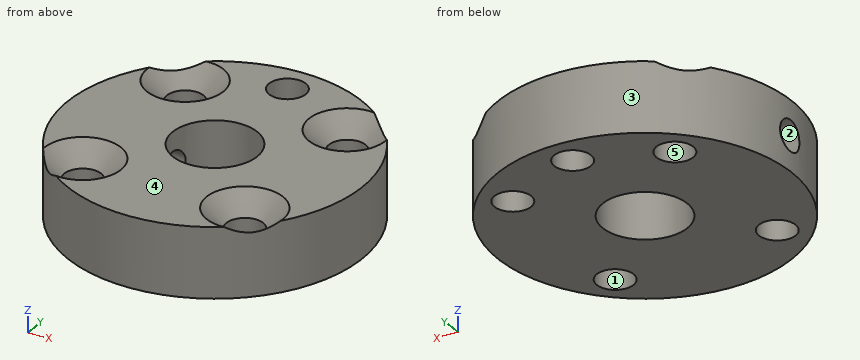
```python
from build123d import *

# Parameters (mm, degrees)
SKETCH2_R                                       = 20
BOSS_EXTRUDE1_DEPTH                             = 9.5
CSK_FOR_M5_FLAT_HEAD_MACHINE_SCREW1_D           = 5
CSK_FOR_M5_FLAT_HEAD_MACHINE_SCREW1_CSINK_D     = 10.4
CSK_FOR_M5_FLAT_HEAD_MACHINE_SCREW1_CSINK_ANGLE = 90
SKETCH5_R                                       = 2.5
CUT_EXTRUDE1_DEPTH                              = 30.837057662
SKETCH6_R                                       = 5.75
CUT_EXTRUDE2_DEPTH                              = 30.837057662
SKETCH8_R                                       = 2.1
CUT_EXTRUDE3_DEPTH                              = 30.837057662


with BuildPart() as part:
    # Sketch2 → Boss-Extrude1 (new body)
    with BuildSketch(Plane.XY):
        Circle(SKETCH2_R)
    extrude(amount=BOSS_EXTRUDE1_DEPTH)

    # CSK for M5 Flat Head Machine Screw1 (through all)
    with Locations(Plane.XY.offset(9.5)):
        with Locations((-11.136931804, 11.136931804), (11.136931804, 11.136931804), (11.136931804, -11.136931804), (-11.136931804, -11.136931804)):
            CounterSinkHole(CSK_FOR_M5_FLAT_HEAD_MACHINE_SCREW1_D / 2, CSK_FOR_M5_FLAT_HEAD_MACHINE_SCREW1_CSINK_D / 2, counter_sink_angle=CSK_FOR_M5_FLAT_HEAD_MACHINE_SCREW1_CSINK_ANGLE)

    # Sketch5 → Cut-Extrude1 (cut, through all)
    with BuildSketch(Plane.XY.offset(9.5)):
        with Locations((0, 15.75)):
            Circle(SKETCH5_R)
    extrude(amount=-CUT_EXTRUDE1_DEPTH, mode=Mode.SUBTRACT)

    # Sketch6 → Cut-Extrude2 (cut, through all)
    with BuildSketch(Plane.XY.offset(9.5)):
        Circle(SKETCH6_R)
    extrude(amount=-CUT_EXTRUDE2_DEPTH, mode=Mode.SUBTRACT)

    # Sketch8 → Cut-Extrude3 (cut, through all)
    with BuildSketch(Plane(origin=(0, 0, 0), x_dir=(0, 0, -1), z_dir=(1, 0, 0))):
        with Locations((-4.75, 0)):
            Circle(SKETCH8_R)
    extrude(amount=-CUT_EXTRUDE3_DEPTH, mode=Mode.SUBTRACT)


solid = part.part
```
Design review of the part built by this model. Coordinates are the model's own, in mm. Face numbers are marked on the shaded views. A direction names the side the tool comes from. Coordinates: 2 decimals unless noted, no trailing zeros. Loops run counter-clockwise (first coordinate to the right, second up) from the corner with the lowest first, then second, coordinate; pieces in that order, holes last.
Q1. We need section D-D on x = 4.5. State the section outline as (y, z) points, and give its area (3 significant figures).
Reported:
outline: (-19.49, 0) - (-3.58, 0) - (-3.58, 9.5) - (-19.49, 9.5) - close; (3.58, 0) - (19.49, 0) - (19.49, 9.5) - (3.58, 9.5) - close
area: 302 mm2
Q2. To check wall thickness, follow line 1 (Y direction, x = 0, z = 3); line 2 (X direction, y = -11, z = 6); line 3 (X direction, y = -13, z = 1.5). State the ranges of each line that lie inside material, in increasing order.
Reported:
line 1: y = -20 to -5.75, 5.75 to 13.25, 18.25 to 20
line 2: x = -16.7 to -13.63, -8.64 to 8.64, 13.63 to 16.7
line 3: x = -15.2 to -12.8, -9.47 to 9.47, 12.8 to 15.2
Q3. Tool access review of the marked faces 1 and 2: name each direction out of +Z, -Z, +X, -X, +Y, -Y from which nothing blocks a thin tool from reaching the whole face with its end or side.
Reported:
face 1: +Z, -Z
face 2: -X
Q4. We need section B-B on x = 0. State the section outline as (y, z) points.
Reported:
outline: (-20, 0) - (-5.75, 0) - (-5.75, 9.5) - (-20, 9.5) - close; (5.75, 0) - (13.25, 0) - (13.25, 9.5) - (5.75, 9.5) - close; (18.25, 0) - (20, 0) - (20, 9.5) - (18.25, 9.5) - close
Q5. We need section C-C on z = 4.75. State the section outline as (x, y) points.
Reported:
outline: (-19.89, -2.1) arc R20 ccw (long way) to (-19.89, 2.1) - (-5.35, 2.1) arc R5.75 cw (long way) to (-5.35, -2.1) - close; hole circle Ø5 at (-11.14, -11.14); hole circle Ø5 at (-11.14, 11.14); hole circle Ø5 at (0, 15.75); hole circle Ø5 at (11.14, -11.14); hole circle Ø5 at (11.14, 11.14)
Q6. For pin 1 (10.5 mm diameter, centred on x = 0, y = 0, fed in from +Z); pin 2 (8 mm diameter, centred on x = 11.14, y = 11.14, fed in from +Z); pin 3 (6 mm diameter, centred on x = -11.14, y = -11.14, fed in from +Z); pin 4 (1 mm diameter, centred on y = -7.5, z = 6.5, fed in from +X) (3 decimals), all flat-tipped, find the tip position at first contact; note any pin that passes through.
Reported:
pin 1: passes through
pin 2: stops at z = 8.3
pin 3: stops at z = 7.3
pin 4: stops at x = 18.735
Q7. We need section A-A on y = 0. State the section outline as (x, z) points.
Reported:
outline: (-20, 0) - (-5.75, 0) - (-5.75, 2.65) - (-20, 2.65) - close; (-20, 6.85) - (-5.75, 6.85) - (-5.75, 9.5) - (-20, 9.5) - close; (5.75, 0) - (20, 0) - (20, 9.5) - (5.75, 9.5) - close
Q8. The part is to be moulded in two halves that separate along Y. For the marked faces 3, 4 and 5, say which applies: +Y half, -Y half, draft (parallel to the pull), parting line (faces both ways), or undercut.
Reported:
face 3: parting line
face 4: draft
face 5: undercut
